Part model, mm, in its own coordinate system. A direction names the side the tool comes from. Coordinates: 2 decimals unless noted, no trailing zeros. Loops run counter-clockwise (first coordinate to the right, second up) from the corner with the lowest first, then second, coordinate; pieces in that order, holes last.
```python
from build123d import *

# Parameters (mm, degrees)
SKETCH_W     = 10
SKETCH_H     = 10
PAD_DEPTH    = 50
POCKET_DEPTH = 50.001


with BuildPart() as part:
    # Sketch → Pad (new body)
    with BuildSketch(Plane.YZ):
        with Locations((5, 5)):
            Rectangle(SKETCH_W, SKETCH_H)
    extrude(amount=PAD_DEPTH)

    # Sketch001 (on Face5 of Pad) → Pocket (cut, through all)
    with BuildSketch(Plane(origin=(0, 0, 0), x_dir=(0, 1, 0), z_dir=(-1, 0, 0))):
        with BuildLine():
            Line((8.5, -10), (8.5, -3.5))
            ThreePointArc((8.5, -3.5), (7.914214, -2.085786), (6.5, -1.5))
            Line((6.5, -1.5), (3.5, -1.5))
            ThreePointArc((3.5, -1.5), (2.085786, -2.085786), (1.5, -3.5))
            Line((1.5, -3.5), (1.5, -10))
            Line((1.5, -10), (8.5, -10))
        make_face()
    extrude(amount=-POCKET_DEPTH, mode=Mode.SUBTRACT)


solid = part.part
```
Q1. Saw through at A-A (z = 9.5). List the corners of the cut face in (x, y).
Q2. Drop a flat-ended pin along its axis: P1, Ø3.5, axis at x = 31.5, y = 5.5, coming from the +Z side. Give the stop position or say it passes through.
Q3. Tool access for faces 4 (the flat face through (25, 9, 10)), 5 (the flat face through (25, 5, 1.5)): list every direction of +Z, -Z, +X, -X, +Y, -Y with a clear straight run to the whole face (end or side of a thin tool).
Q4. Mould opens along Y. For faces 1 (the cylindrical face through (24.65, 7.93, 2.1)), 2 (the flat face through (25, 10, 5)), 3 (the flat face through (50, 5, 1)) say: released by +Y, released by -Y, zero draft, split by the parting line, or undercut.
Q5. Probe line 1 (Y direction, x = 24.5, z = 5.5); line 2 (Z direction, x = 6.5, y = 6.5); line 3 (Y direction, x = 36, z = 2). List the from-to ranges inside material, lowest first.
Q6. Saw through at B-B (x = 8). List the corners of the cut face in (y, z).
Q7. Saw through at D-D (y = 5). List the corners of the cut face in (x, z), plus the area to 3 significant figures.
Q8. Saw through at C-C (z = 2.25). List the corners of the cut face in (x, y), plus the area to 3 significant figures.
Checked values:
1. outline: (0, 0) - (50, 0) - (50, 1.5) - (0, 1.5) - close; (0, 8.5) - (50, 8.5) - (50, 10) - (0, 10) - close
2. P1: stops at z = 1.65
3. face 4: +Z, +X, -X, +Y, -Y
3. face 5: +Z, +X, -X
4. face 1: undercut
4. face 2: released by +Y
4. face 3: zero draft
5. line 1: y = 0 to 1.5, 8.5 to 10
5. line 2: z = 0 to 1.5
5. line 3: y = 0 to 2.18, 7.82 to 10
6. outline: (0, 0) - (10, 0) - (10, 10) - (8.5, 10) - (8.5, 3.5) arc R2 cw to (6.5, 1.5) - (3.5, 1.5) arc R2 cw to (1.5, 3.5) - (1.5, 10) - (0, 10) - close
7. outline: (0, 0) - (50, 0) - (50, 1.5) - (0, 1.5) - close
7. area: 75.0 mm2
8. outline: (0, 0) - (50, 0) - (50, 1.94) - (0, 1.94) - close; (0, 8.06) - (50, 8.06) - (50, 10) - (0, 10) - close
8. area: 194 mm2
